```python
from build123d import *


with BuildPart() as part:
    # SealProfileS → SealProfile (revolve)
    with BuildSketch(Plane.XY, mode=Mode.PRIVATE) as sealprofile_sk:
        Polygon((5, 0), (5, 1.8), (5.8, 1.8), (5.9, 1), (6.1, 1), (6.6, 1.8), (6.8, 1.8), (7, 1.3), (6.7, 0), align=None)
    revolve(sealprofile_sk.sketch.rotate(Axis((0, 0, 0), (0, 1, 0)), 90), axis=Axis((0, 0, 0), (0, 1, 0)))


solid = part.part
```
Geometry: final body of the model. Coordinates: model frame, mm. Coordinates: 2 decimals unless noted, no trailing zeros. Write each loop counter-clockwise with the first axis right and the second up, starting at its lowest first coordinate (ties: lowest second). Pieces come first, ordered by that corner, then holes. Notation, with made-up numbers: M -3,17.5 L 31,17.5 A18 ccw 31,27.5 Z; hole C 1.25,-40 d2. An arc over 180 degrees is marked long. Answer as CSV lines item,"result". Start each with the question number.
Q1. Cut plane A-A on x = 0. Return the cut outline in (y, z).
Q2. Line query: line 1 (Z direction, x = -3, y = 1.25); line 2 (Z direction, x = -2.5, y = 1.55); line 3 (X direction, y = 1.35, z = 0). Output: solid intervals per line, ascending. Write a range as from..to.
Q3. Cut plane C-C on y = 0.3. Return the cut outline in (x, z).
Q4. Mould query, pull axis Z, two halves, no side actions, for faces 1 (the cylindrical face through (0, 1, 5)), 2 (the flat face through (-5, 1.8, 2)). Classes: released by +Z, released by -Z, zero draft, split by the parting line, or undercut.
Q5. Pin query (flat end, axial travel): P1, Ø5, axis at x = -3.5, z = -2.5, coming from the -Y side. Return the tip coordinate at first contact, or that it passes through.
Q6. Cut plane B-B on z = 0. Return the cut outline in (x, y).
Findings below:
1,outline,"M 0,-6.7 L 1.3,-7 L 1.8,-6.8 L 1.8,-6.6 L 1,-6.1 L 1,-5.9 L 1.8,-5.8 L 1.8,-5 L 0,-5 Z; M 0,5 L 1.8,5 L 1.8,5.8 L 1,5.9 L 1,6.1 L 1.8,6.6 L 1.8,6.8 L 1.3,7 L 0,6.7 Z"
2,line 1,"z = -6.31..-5.49, -5.04..-4, 4..5.04, 5.49..6.31"
2,line 2,"z = -6.43..-5.94, -5.27..-4.33, 4.33..5.27, 5.94..6.43"
2,line 3,"x = -6.98..-6.32, -5.86..-5, 5..5.86, 6.32..6.98"
3,outline,"C 0,0 d13.54; hole C 0,0 d10"
4,face 1,"undercut"
4,face 2,"zero draft"
5,P1,"stops at y = 0"
6,outline,"M -7,1.3 L -6.7,0 L -5,0 L -5,1.8 L -5.8,1.8 L -5.9,1 L -6.1,1 L -6.6,1.8 L -6.8,1.8 Z; M 5,0 L 6.7,0 L 7,1.3 L 6.8,1.8 L 6.6,1.8 L 6.1,1 L 5.9,1 L 5.8,1.8 L 5,1.8 Z"
